from build123d import *

# Parameters (mm, degrees)
SKETCH1_W          = 40
SKETCH1_H          = 45
BASE_DEPTH         = 6
WIRE_GROOVES_DEPTH = 50.608467019


with BuildPart() as part:
    # Sketch1 → Base (new body)
    with BuildSketch(Plane.XY):
        Rectangle(SKETCH1_W, SKETCH1_H)
    extrude(amount=BASE_DEPTH)

    # Sketch2 → Wire Grooves (cut, through all)
    with BuildSketch(Plane(origin=(0, 22.5, 0), x_dir=(1, 0, 0), z_dir=(0, 1, 0))):
        with BuildLine():
            Line((-13.8, 0), (-10, 0))
            ThreePointArc((-10, 0), (-11.9, -1.9), (-13.8, 0))
        make_face()
        with BuildLine():
            Line((13.8, 0), (10, 0))
            ThreePointArc((10, 0), (11.9, -1.9), (13.8, 0))
        make_face()
    extrude(amount=-WIRE_GROOVES_DEPTH, mode=Mode.SUBTRACT)


solid = part.part
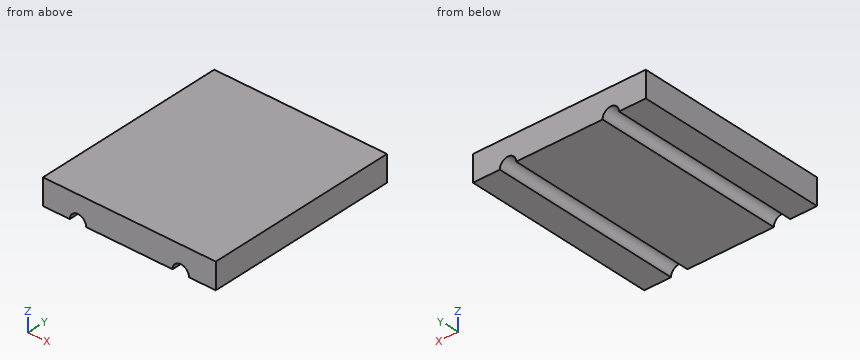
Verification items for the finished model (mm, model axes). Give positions to 0.01 mm unless a question says otherwise; leave off trailing zeros. Loops run counter-clockwise (first coordinate to the right, second up) from the corner with the lowest first, then second, coordinate; pieces in that order, holes last.
1) Thickness scan on line 1 along X through (y, z) = (1.5, 1.15); line 2 along X through (y, z) = (-7, 0.85); line 3 along Z through (x, y) = (12, 5.5). Record the ranges inside material, lowest first.
2) Depth check by flat-ended pin: pin 1 Ø3 at (x, y) = (12.5, 7.5) entering from -Z. Enter the tip coordinate at first touch or a pass-through.
3) Sectioned sample at A-A, the plane z = 0.7. Enter the section's corners in (x, y), then the cut area to 3 significant figures.
4) Sectioned sample at C-C, the plane x = -11.9. Enter the section's corners in (y, z).
5) Sectioned sample at B-B, the plane y = 18. Enter the section's corners in (x, z), then the cut area to 3 significant figures.
Answers:
1. line 1: x = -20 to -13.41, -10.39 to 10.39, 13.41 to 20
1. line 2: x = -20 to -13.6, -10.2 to 10.2, 13.6 to 20
1. line 3: z = 1.9 to 6
2. pin 1: stops at z = 0
3. outline: (-20, -22.5) - (-13.67, -22.5) - (-13.67, 22.5) - (-20, 22.5) - close; (-10.13, -22.5) - (10.13, -22.5) - (10.13, 22.5) - (-10.13, 22.5) - close; (13.67, -22.5) - (20, -22.5) - (20, 22.5) - (13.67, 22.5) - close
3. area: 1,480 mm2
4. outline: (-22.5, 1.9) - (22.5, 1.9) - (22.5, 6) - (-22.5, 6) - close
5. outline: (-20, 0) - (-13.8, 0) arc R1.9 cw to (-10, 0) - (10, 0) arc R1.9 cw to (13.8, 0) - (20, 0) - (20, 6) - (-20, 6) - close
5. area: 229 mm2
